from build123d import *

# Parameters (mm, degrees)
F0_W     = 127
F0_H     = 304.8
F1_DEPTH = 19.05
F3_DEPTH = 6.35
F4_R     = 3.175
F5_DEPTH = 12.701
F6_W     = 25.4
F6_H     = 9.525
F7_DEPTH = 127.001
F8_W     = 19.05
F8_H     = 76.2
F9_DEPTH = 9.525
F10_R    = 6.35


with BuildPart() as f1:
    # F0 (on Front) → F1 (new body)
    with BuildSketch(Plane.XZ):
        Rectangle(F0_W, F0_H)
    extrude(amount=F1_DEPTH)

    # F2 (on face) → F3 (cut)
    with BuildSketch(Plane(origin=(0, 0, 0), x_dir=(-1, 0, 0), z_dir=(0, 1, 0))):
        with BuildLine():
            Line((12.7, 114.3), (12.7, 152.4))
            ThreePointArc((12.7, 152.4), (0, 165.1), (-12.7, 152.4))
            Line((-12.7, 152.4), (-12.7, 114.3))
            ThreePointArc((-12.7, 114.3), (0, 101.6), (12.7, 114.3))
        make_face()
    extrude(amount=-F3_DEPTH, mode=Mode.SUBTRACT)

    # F4 (on face) → F5 (cut, through all)
    with BuildSketch(Plane(origin=(0, -6.35, 0), x_dir=(-1, 0, 0), z_dir=(0, 1, 0))):
        with Locations((0, 114.3)):
            Circle(F4_R)
        with Locations((0, 139.7)):
            Circle(F4_R)
    extrude(amount=-F5_DEPTH, mode=Mode.SUBTRACT)

    # F6 (on face) → F7 (cut, through all)
    with BuildSketch(Plane(origin=(-63.5, 0, 0), x_dir=(0, -1, 0), z_dir=(-1, 0, 0))):
        with Locations((22.225, -147.6375)):
            Rectangle(F6_W, F6_H)
    extrude(amount=-F7_DEPTH, mode=Mode.SUBTRACT)

    # F8 (on face) → F9 (cut)
    with BuildSketch(Plane.XZ.offset(19.05)):
        with Locations((0, -104.775)):
            Rectangle(F8_W, F8_H)
    extrude(amount=-F9_DEPTH, mode=Mode.SUBTRACT)

    # F10
    f10_edges = [f1.edges().sort_by_distance(p)[0] for p in [
        (-9.525, -14.2875, -66.675),
        (9.525, -14.2875, -66.675),
    ]]
    fillet(f10_edges, radius=F10_R)


with BuildPart() as f11_1:
    # F11: copy of F1
    add(f1.part)


solid = f1.part
Design review of the part built by this model. Coordinates are the model's own, in mm. A direction names the side the tool comes from. Coordinates: 2 decimals unless noted, no trailing zeros. Write each loop counter-clockwise with the first axis right and the second up, starting at its lowest first coordinate (ties: lowest second). Pieces come first, ordered by that corner, then holes. Notation, with made-up numbers: (-17.5, 57.5) - (20.5, 57.5) arc R22 ccw to (20.5, 82.5) - close; hole circle Ø9 at (55, 40). An arc over 180 degrees is marked (long way). Use one line per item in the form item = value.
Q1. Consider section B-B (x = 0). Write out the cut boundary in (y, z) (3 decimals), plus the area to 3 significant figures.
Taken from the geometry:
outline = (-19.05, -66.675) - (-9.525, -66.675) - (-9.525, -152.4) - (0, -152.4) - (0, 101.6) - (-6.35, 101.6) - (-6.35, 111.125) - (-19.05, 111.125) - close; (-19.05, 117.475) - (-6.35, 117.475) - (-6.35, 136.525) - (-19.05, 136.525) - close; (-19.05, 142.875) - (-6.35, 142.875) - (-6.35, 152.4) - (-19.05, 152.4) - close
area = 4,510 mm^2
Q2. Consider section A-A (z = 139.7). Write out the cut boundary in (x, y) (3 decimals).
Taken from the geometry:
outline = (-63.5, -19.05) - (-3.175, -19.05) - (-3.175, -6.35) - (-12.7, -6.35) - (-12.7, 0) - (-63.5, 0) - close; (3.175, -19.05) - (63.5, -19.05) - (63.5, 0) - (12.7, 0) - (12.7, -6.35) - (3.175, -6.35) - close
Q3. For probe 1 along Z at (x, y) = (0, -9) (3 decimals); probe 2 along Z at (x, y) = (0, -10) (3 decimals); probe 3 along X at (y, z) = (-16.25, -122.5) (3 decimals), list the stretches that pass through material, from the lowest coordinate up.
Taken from the geometry:
probe_1 = -152.4 to 111.125, 117.475 to 136.525, 142.875 to 152.4
probe_2 = -66.675 to 111.125, 117.475 to 136.525, 142.875 to 152.4
probe_3 = -63.5 to -9.525, 9.525 to 63.5
Q4. Consider section C-C (x = -28.5). Write out the cut boundary in (y, z) (3 decimals).
Taken from the geometry:
outline = (-19.05, -142.875) - (-9.525, -142.875) - (-9.525, -152.4) - (0, -152.4) - (0, 152.4) - (-19.05, 152.4) - close
Q5. Machinability: for faces 1 (the cylindrical face through (0.279, -3.131, 101.603)), 2 (the cylindrical face through (0.69, -12.61, 111.2)), 3 (the flat face through (36, -14, -142.875)), 4 (the cylindrical face through (7.71, -14.22, -68.58)), which of the approach directions +Z, -Z, +X, -X, +Y, -Y give a long, thin tool a straight path to every point of the face, cutting with its end or side? Answer none if there is none.
Taken from the geometry:
face_1 = +Z, +Y
face_2 = +Y, -Y
face_3 = -Z, +X, -X, -Y
face_4 = -Z, -Y
Q6. Insertion check: pin 1 Ø5 at (x, z) = (45.5, 118) entering from +Y; pin 2 Ø3 at (x, y) = (44, -16.5) entering from -Z (3 decimals); pin 3 Ø7 at (x, y) = (1.5, -16) entering from -Z. Each pin has a flat end and moves straight along its axis. Give the tip position at first contact, or say it passes through.
Taken from the geometry:
pin_1 = 0
pin_2 = -142.875
pin_3 = -66.94
Q7. The part is to be moulded in two halves that separate along X. For faces 5 (the flat face through (63.5, -9, -2)), 6 (the flat face through (-1, -19.05, 7)), 7 (the cylindrical face through (0.41, -12.61, 142.85)), say which applies: +X half, -X half, draft (parallel to the pull), parting line (faces both ways), or undercut.
Taken from the geometry:
face_5 = +X half
face_6 = draft
face_7 = undercut
